For this review, take the finished solid that the model builds, in its own axes (mm). A direction names the side the tool comes from. Round coordinates to 2 decimals unless told otherwise and drop trailing zeros. Loops run counter-clockwise (first coordinate to the right, second up) from the corner with the lowest first, then second, coordinate; pieces in that order, holes last.
1. Draft analysis for pull direction Z (two halves, no side actions). For faces 4 (the flat face through (-24, 52, 34.925)), 5 (the cylindrical face through (3.645, 96.356, 2.348)), 6 (the flat face through (-4, 82.55, 17)), state which applies: released by +Z, released by -Z, zero draft, split by the parting line, or undercut.
2. Clearance check with flat-ended pins moving along their axes: pin 1 Ø9 at (x, y) = (4.17, 92.39) entering from +Z (3 decimals); pin 2 Ø5 at (x, z) = (-9.5, 28) entering from -Y; pin 3 Ø1 at (y, z) = (82, 24) entering from -X; pin 4 Ø6 at (x, z) = (-73.025, 19.05) entering from -Y. State where each tip first meets the part, or that it passes through.
3. To check wall thickness, follow line 1 along Z through (x, y) = (-2, 97) (1 decimal); line 2 along Z through (x, y) = (-70.5, 24) (3 decimals); line 3 along X through (y, z) = (25, 19). State the ranges of each line that lie inside material, in increasing order.
4. Tool access review of faces 1 (the flat face through (-10, 50.8, 29)), 2 (the flat face through (-42, 19.05, 18)), 3 (the flat face through (1, 88, 4.762)): name each direction out of +Z, -Z, +X, -X, +Y, -Y from which nothing blocks a thin tool from reaching the whole face with its end or side.
5. Consider section A-A on y = 84.5. State the section outline as (x, z) points (1 decimal), then the cut area to 3 significant figures.
6. Consider section B-B on z = 19.05. State the section outline as (x, y) points.
7. Consider section D-D on z = 3. State the section outline as (x, y) points (3 decimals).
8. Consider section C-C on y = 74.5. State the section outline as (x, z) points (1 decimal), then the cut area to 3 significant figures.
from build123d import *

# Parameters (mm, degrees)
SKETCH1_R           = 4
BOSS_EXTRUDE1_DEPTH = 4.7625
SKETCH2_R           = 4
BOSS_EXTRUDE2_DEPTH = 25.4
BOSS_EXTRUDE3_START = 30.1625
SKETCH1_2_R         = 4
BOSS_EXTRUDE3_DEPTH = 4.7625
SKETCH4_W           = 82.55
SKETCH4_H           = 34.925
CUT_EXTRUDE1_DEPTH  = 19.05
SKETCH5_R           = 3.2639
CUT_EXTRUDE2_DEPTH  = 31.75


with BuildPart() as part:
    # Sketch1 → Boss-Extrude1 (new body)
    with BuildSketch(Plane.XY):
        with BuildLine():
            Line((0, 0), (0, 19.05))
            Line((0, 19.05), (13.525460699, 90.621522374))
            ThreePointArc((13.525460699, 90.621522374), (8.613422955, 100.813245135), (-2.573048888, 99.121448653))
            Line((-2.573048888, 99.121448653), (-82.55, 19.05))
            Line((-82.55, 19.05), (-82.55, 0))
            Line((-82.55, 0), (0, 0))
        make_face()
        with Locations((4.166118695, 92.390234401)):
            Circle(SKETCH1_R, mode=Mode.SUBTRACT)
        with Locations((-9.525, 9.525)):
            Circle(SKETCH1_R, mode=Mode.SUBTRACT)
        with Locations((-73.025, 9.525)):
            Circle(SKETCH1_R, mode=Mode.SUBTRACT)
    extrude(amount=BOSS_EXTRUDE1_DEPTH)

    # Sketch2 → Boss-Extrude2 (add)
    with BuildSketch(Plane.XY.offset(4.7625)):
        Polygon((-19.124940493, 82.55), (12.000118566, 82.55), (0, 19.05), (0, 0), (-82.55, 0), (-82.55, 19.05), align=None)
        with Locations((-73.025, 9.525)):
            Circle(SKETCH2_R, mode=Mode.SUBTRACT)
        with Locations((-9.525, 9.525)):
            Circle(SKETCH2_R, mode=Mode.SUBTRACT)
    extrude(amount=BOSS_EXTRUDE2_DEPTH)

    # Sketch1<2> → Boss-Extrude3 (add)
    with BuildSketch(Plane.XY.offset(BOSS_EXTRUDE3_START)):
        with BuildLine():
            Line((0, 0), (0, 19.05))
            Line((0, 19.05), (13.525460699, 90.621522374))
            ThreePointArc((13.525460699, 90.621522374), (8.613422955, 100.813245135), (-2.573048888, 99.121448653))
            Line((-2.573048888, 99.121448653), (-82.55, 19.05))
            Line((-82.55, 19.05), (-82.55, 0))
            Line((-82.55, 0), (0, 0))
        make_face()
        with Locations((4.166118695, 92.390234401)):
            Circle(SKETCH1_2_R, mode=Mode.SUBTRACT)
        with Locations((-9.525, 9.525)):
            Circle(SKETCH1_2_R, mode=Mode.SUBTRACT)
        with Locations((-73.025, 9.525)):
            Circle(SKETCH1_2_R, mode=Mode.SUBTRACT)
    extrude(amount=BOSS_EXTRUDE3_DEPTH)

    # Sketch4 → Cut-Extrude1 (cut)
    with BuildSketch(Plane.XZ):
        with Locations((-41.275, 17.4625)):
            Rectangle(SKETCH4_W, SKETCH4_H)
    extrude(amount=-CUT_EXTRUDE1_DEPTH, mode=Mode.SUBTRACT)

    # Sketch5 → Cut-Extrude2 (cut)
    with BuildSketch(Plane.XZ.offset(-19.05)):
        with Locations((-9.525, 9.525)):
            Circle(SKETCH5_R)
        with Locations((-73.025, 9.525)):
            Circle(SKETCH5_R)
        with Locations((-73.025, 28.575)):
            Circle(SKETCH5_R)
        with Locations((-9.525, 28.575)):
            Circle(SKETCH5_R)
        with Locations((-73.025, 19.05)):
            Circle(SKETCH5_R)
        with Locations((-9.525, 19.05)):
            Circle(SKETCH5_R)
    extrude(amount=-CUT_EXTRUDE2_DEPTH, mode=Mode.SUBTRACT)


solid = part.part
Resolved:
1. face 4: released by +Z
1. face 5: zero draft
1. face 6: undercut
2. pin 1: stops at z = 34.925
2. pin 2: stops at y = 50.8
2. pin 3: stops at x = -20.17
2. pin 4: passes through
3. line 1: z = 0 to 4.8, 30.2 to 34.9
3. line 2: z = 0 to 7.457, 11.593 to 16.982, 21.118 to 26.507, 30.643 to 34.925
3. line 3: x = -76.61 to -76.29, -69.76 to -12.79, -6.26 to 1.12
4. face 1: -Y
4. face 2: +Z, -Z, +X, -X, -Y
4. face 3: +X, -X, +Y
5. outline: (-17.2, 0) - (12.4, 0) - (12.4, 4.8) - (-17.2, 4.8) - close; (-17.2, 30.2) - (12.4, 30.2) - (12.4, 34.9) - (-17.2, 34.9) - close
5. area: 281 mm2
6. outline: (-82.55, 19.05) - (-76.29, 19.05) - (-76.29, 25.32) - close; (-69.76, 19.05) - (-12.79, 19.05) - (-12.79, 50.8) - (-6.26, 50.8) - (-6.26, 19.05) - (0, 19.05) - (12, 82.55) - (-19.12, 82.55) - (-69.76, 31.85) - close
7. outline: (-82.55, 19.05) - (0, 19.05) - (13.525, 90.622) arc R9.525 ccw to (-2.573, 99.121) - close; hole circle Ø8 at (4.166, 92.39)
8. outline: (-27.2, 0) - (10.5, 0) - (10.5, 34.9) - (-27.2, 34.9) - close
8. area: 1,310 mm2
